Input: part model. Units: mm. Frame: model coordinates. A direction names the side the tool comes from. Coordinates: 2 decimals unless noted, no trailing zeros. Loops run counter-clockwise (first coordinate to the right, second up) from the corner with the lowest first, then second, coordinate; pieces in that order, holes last. Notation, with made-up numbers: M 80,76.5 L 95,76.5 A15 ccw 95,94.5 Z; hole C 2.5,15.25 d4. An arc over 180 degrees is marked long. Use a Markdown table: item, result. Add a question column.
1. Pin query (flat end, axial travel): pin 1 (1.2 mm diameter, centred on x = 20.5, y = 3, fed in from +Z); pin 2 (1.3 mm diameter, centred on y = -1, z = 2, fed in from +X); pin 3 (2 mm diameter, centred on x = 20, y = 2, fed in from -Z). Return the tip coordinate at first contact, or that it passes through.
2. Section A-A on z = -2.5. Output: boundary loops of the cut face in (x, y), then the cut area to 3 significant figures.
3. Set-up query: faces 1 (the flat face through (19, 2, 3.5)), 2 (the flat face through (19, 2, -3.5)), 3 (the flat face through (22, 0, 0)). Return all of +Z, -Z, +X, -X, +Y, -Y with unobstructed straight access to the full face (end or side cutting, diameter ignored); none if empty.
4. Section C-C on x = 2. Output: boundary loops of the cut face in (y, z).
5. Line query: L1, parallel to Y at x = -1.5, z = 3.5; L2, parallel to Z at x = 20, y = 0.6; L3, parallel to X at y = -0.3, z = 2.25. Output: solid intervals per line, ascending. Write a range as [from, to].
6. Section B-B on y = 1.15. Output: boundary loops of the cut face in (x, z).
```python
from build123d import *

# Parameters (mm, degrees)
ESBO_O1_W                = 42.5
ESBO_O1_H                = 18
RESSALTO_EXTRUS_O1_DEPTH = 1.6
RESSALTO_EXTRUS_O2_DEPTH = 4


with BuildPart() as part:
    # Esboço1 → Ressalto-extrusão1 (new body)
    with BuildSketch(Plane(origin=(0, 0, 0), x_dir=(1, 0, 0), z_dir=(0, 1, 0))):
        Rectangle(ESBO_O1_W, ESBO_O1_H)
    extrude(amount=-RESSALTO_EXTRUS_O1_DEPTH)

    # Esboço2 → Ressalto-extrusão2 (add)
    with BuildSketch(Plane(origin=(0, 0, 0), x_dir=(1, 0, 0), z_dir=(0, 1, 0))):
        Polygon((21.25, 3.5), (23.25, 3.5), (23.25, -3.5), (21.25, -3.5), (14.25, -3.5), (14.25, 3.5), align=None)
    extrude(amount=RESSALTO_EXTRUS_O2_DEPTH)


solid = part.part
```
Answers below:
| question | item | result |
|---|---|---|
| 1 | pin 1 | stops at z = 3.5 |
| 1 | pin 2 | stops at x = 21.25 |
| 1 | pin 3 | stops at z = -3.5 |
| 2 | outline | M -21.25,-1.6 L 21.25,-1.6 L 21.25,0 L 23.25,0 L 23.25,4 L 14.25,4 L 14.25,0 L -21.25,0 Z |
| 2 | area | 104 mm² |
| 3 | face 1 | +Z, +X, -X, +Y |
| 3 | face 2 | -Z, +X, -X, +Y |
| 3 | face 3 | +Z, -Z, +X, -Y |
| 4 | outline | M -1.6,-9 L 0,-9 L 0,9 L -1.6,9 Z |
| 5 | L1 | y = [-1.6, 0] |
| 5 | L2 | z = [-3.5, 3.5] |
| 5 | L3 | x = [-21.25, 21.25] |
| 6 | outline | M 14.25,-3.5 L 23.25,-3.5 L 23.25,3.5 L 14.25,3.5 Z |
